Geometry check sheet. Reference: the model listing, model coordinates, mm. A direction names the side the tool comes from. Round coordinates to 2 decimals unless told otherwise and drop trailing zeros.
(1) Draft check along Z on faces 5 (the face through (71.83, 15.01, 37.44)), 6 (the face through (-65.023, 15.014, -61.603)), 7 (the face through (13, 16, 74)). Enter one of: pulls with the +Z half, pulls with the -Z half, needs draft (parallel to the pull), parting line crosses it, or undercut.
(2) Set-up check for faces 1 (the face through (-66, 14, 40)), 2 (the face through (19.05, 15.01, 78.73)), 3 (the face through (-25.296, 18.986, -16.128)), 4 (the face through (75.2, 15, -30.1)): record each of +Z, -Z, +X, -X, +Y, -Y from which the full face is reachable in a straight line by a thin tool's end or side.
(3) Thickness scan on L1, parallel to Y at x = 48.5, z = 63; L2, parallel to X at y = 18.75, z = 10; L3, parallel to Z at x = 8, y = 16.75. Record the ranges inside material, lowest first.
(4) Gauge pin test, flat ends, axial feed: P1, Ø5, axis at x = 48, z = -13, coming from the -Y side; P2, Ø3.5, axis at x = -79.11, z = 31.86, coming from the +Y side; P3, Ø5, axis at x = 27.73, z = -80.65, coming from the -Y side. Record the tip position at first contact, or that the pin passes through.
from build123d import *

# Parameters (mm, degrees)
SKETCH2_R           = 1.5
BOSS_EXTRUDE1_DEPTH = 2
CIRPATTERN1_COUNT   = 11


with BuildPart() as part:
    # Sketch1 → Revolve2 (revolve)
    with BuildSketch(Plane.XY, mode=Mode.PRIVATE) as revolve2_sk:
        with BuildLine():
            ThreePointArc((34.328340107, 16.866562419), (48.522419142, 11.000585737), (63.75, 9))
            Line((63.75, 9), (75, 9))
            Line((75, 9), (76, 9))
            Line((76, 9), (76, 14))
            Line((76, 14), (81, 14))
            Line((81, 14), (81, 16))
            Line((81, 16), (74, 16))
            ThreePointArc((74, 16), (71.148866911, 15.34166622), (68.875, 13.499957088))
            ThreePointArc((68.875, 13.499957088), (66.601133089, 11.658247956), (63.75, 10.999914176))
            ThreePointArc((63.75, 10.999914176), (49.038996589, 12.932632438), (35.32643469, 18.599612884))
            ThreePointArc((35.32643469, 18.599612884), (32.756692767, 19.655344367), (30, 20))
            Line((30, 20), (30, 18))
            ThreePointArc((30, 18), (32.240109584, 17.72327699), (34.328340107, 16.866562419))
        make_face()
    revolve(revolve2_sk.sketch.rotate(Axis((0, -11, 0), (0, 1, 0)), 90), axis=Axis((0, -11, 0), (0, 1, 0)))

    # Sketch2 → Boss-Extrude1 (add)
    with BuildSketch(Plane(origin=(0, 16, 0), x_dir=(1, 0, 0), z_dir=(0, 1, 0))):
        with BuildLine():
            ThreePointArc((69.296531703, 49.288508752), (67.592037892, 46.777022023), (68.141536159, 43.791906214))
            ThreePointArc((68.141536159, 43.791906214), (63.565042795, 50.204435407), (58.387245806, 56.142047765))
            ThreePointArc((58.387245806, 56.142047765), (61.16383943, 54.915918657), (64.001886983, 55.992185739))
            ThreePointArc((64.001886983, 55.992185739), (70.29195078, 55.51742825), (69.296531703, 49.288508752))
        make_face()
        with Locations(Location((66.928496787, 52.860931829, 0), (0, 0, 270))):
            Circle(SKETCH2_R, mode=Mode.SUBTRACT)
    boss_extrude1 = extrude(amount=-BOSS_EXTRUDE1_DEPTH)

    # CirPattern1: Boss-Extrude1 ×11 about axis, 1 skipped
    cirpattern1_axis = Axis((0, 0, 0), (0, -1, 0))
    add([boss_extrude1.rotate(cirpattern1_axis, i * 360 / CIRPATTERN1_COUNT) for i in range(1, CIRPATTERN1_COUNT) if i not in (2,)])


solid = part.part
Found:
1. face 5: pulls with the +Z half
1. face 6: undercut
1. face 7: needs draft
2. face 1: -Y
2. face 2: +Z, +Y, -Y
2. face 3: +Y, -Y
2. face 4: +X, +Y, -Y
3. L1: y = 14 to 16
3. L2: x = -33.6 to -28.28, 28.28 to 33.6
3. L3: z = -37.98 to -33.59, 33.59 to 37.98
4. P1: stops at y = 10.14
4. P2: stops at y = 16
4. P3: stops at y = 14
